Could you check a few things on this model? Use its own coordinates, in mm. Give positions to 0.01 mm unless a question says otherwise; leave off trailing zeros. Order: outer loops, then holes, each group sorted by start corner. A loop starts at its lowest first (then second) coordinate and runs counter-clockwise, first axis right, second up.
from build123d import *

# Parameters (mm, degrees)
SKETCH_1_R            = 3
SKETCH_1_R_2          = 7.5
SKETCH_1_R_3          = 6
EXTRUDE_1_DEPTH       = 4
CUT_EXTRUDE_START     = -10
CUT_EXTRUDE_2_DEPTH   = 10
CHAMFER_START         = -90.054290201
CHAMFER_2_OUTLINE_W   = 9.93243638
CHAMFER_2_OUTLINE_H   = 4
CHAMFER_2_DEPTH       = 0.082131492
CHAMFER_START_2       = -89.972158709
CHAMFER_2_2_OUTLINE_W = 9.93243638
CHAMFER_2_2_OUTLINE_H = 4
CHAMFER_2_2_DEPTH     = 1.179418362
FILLET_4_R            = 15
FILLET_5_R            = 10
CUT_EXTRUDE_6_DEPTH   = 10
FILLET_8_R            = 3


with BuildPart() as part:
    # 草图1 → 凸台-拉伸1 (new body)
    with BuildSketch(Plane.XY):
        with BuildLine():
            Line((-47.486974837, 85.838147942), (-18.140882386, -2.213296441))
            ThreePointArc((-18.140882386, -2.213296441), (-15.593099371, -5.678603485), (-11.5, -7))
            Line((-11.5, -7), (11.5, -7))
            ThreePointArc((11.5, -7), (16.545894038, -4.851695926), (18.494612442, 0.274584754))
            Line((18.494612442, 0.274584754), (14.988455233, 89.588395901))
            ThreePointArc((14.988455233, 89.588395901), (9.660960601, 100.474573642), (-1.973684211, 103.869585423))
            Line((-1.973684211, 103.869585423), (-39.315789474, 98.913056948))
            ThreePointArc((-39.315789474, 98.913056948), (-46.480167485, 94.299694277), (-47.486974837, 85.838147942))
        make_face()
        with Locations((11.5, 0)):
            Circle(SKETCH_1_R, mode=Mode.SUBTRACT)
        with Locations((-11.5, 0)):
            Circle(SKETCH_1_R, mode=Mode.SUBTRACT)
        with Locations((0, 89)):
            Circle(SKETCH_1_R_2, mode=Mode.SUBTRACT)
        with Locations((-38, 89)):
            Circle(SKETCH_1_R_3, mode=Mode.SUBTRACT)
    extrude(amount=EXTRUDE_1_DEPTH)

    # 草图3 → 切除-拉伸2 (cut)
    with BuildSketch(Plane.XY.offset(4).offset(CUT_EXTRUDE_START)):
        with BuildLine():
            Line((-30.07293559, 95.096035584), (-12.403974557, 97.441289229))
            ThreePointArc((-12.403974557, 97.441289229), (-8.018810771, 101.681191682), (-2.308312161, 103.825169261))
            Line((-2.308312161, 103.825169261), (-39.315789474, 98.913056948))
            ThreePointArc((-39.315789474, 98.913056948), (-34.182978636, 98.242853883), (-30.07293559, 95.096035584))
        make_face()
    extrude(amount=CUT_EXTRUDE_2_DEPTH, mode=Mode.SUBTRACT)

    # 倒角1
    # the kernel refuses this chamfer: 10 mm, written as the material it adds along each edge
    with BuildSketch(Plane(origin=(-30.07293559, 95.096035584, 0), x_dir=(-0.7655170404951253, 0.6434156205063604, 0), z_dir=(0, 0, 1))) as chamfer_1_piece_1:
        with BuildLine():
            Line((4.638446898, 0.2), (-5.12937843, -5.439456583))
            Line((-5.12937843, -5.439456583), (-5.277087929, -5.304616293))
            ThreePointArc((-5.277087929, -5.304616293), (-2.667716566, -2.625677211), (-0.147709499, 0.13484029))
            Line((-0.147709499, 0.13484029), (0.042920367, 0.195340324))
            ThreePointArc((0.042920367, 0.195340324), (2.321577959, -0.03141118), (4.595526531, 0.395340324))
            Line((4.595526531, 0.395340324), (4.638446898, 0.2))
        make_face()
    extrude(amount=4)

    # 倒角2: read off the stored shape, not the designer's step
    # 倒角2 outline → 倒角2 (cut)
    with BuildSketch(Plane(origin=(0, 0, 0), x_dir=(0.8432639594677478, 0.5374996694536441, 0), z_dir=(0.537499669453644, -0.8432639594677479, 0)).offset(CHAMFER_START)):
        with Locations((44.438996955, 2)):
            Rectangle(CHAMFER_2_OUTLINE_W, CHAMFER_2_OUTLINE_H)
    extrude(amount=CHAMFER_2_DEPTH, mode=Mode.SUBTRACT)

    # Chamfer 2 2 outline → Chamfer 2 2 (add)
    with BuildSketch(Plane(origin=(0, 0, 0), x_dir=(0.8432639594677478, 0.5374996694536441, 0), z_dir=(0.537499669453644, -0.8432639594677479, 0)).offset(CHAMFER_START_2)):
        with Locations((44.438996955, 2)):
            Rectangle(CHAMFER_2_2_OUTLINE_W, CHAMFER_2_2_OUTLINE_H)
    extrude(amount=CHAMFER_2_2_DEPTH)

    # 圆角4
    fillet_4_edges = [part.edges().sort_by_distance(p)[0] for p in [
        (-23.040343668, 96.029492385, 2),
        (-33.358562851, 97.857599065, 2),
        (-15.074033854, 97.086884333, 2),
    ]]
    fillet(fillet_4_edges, radius=FILLET_4_R)

    # 圆角5
    fillet_5_edges = [part.edges().sort_by_distance(p)[0] for p in [
        (-6.698368225, 102.425565605, 2),
    ]]
    fillet(fillet_5_edges, radius=FILLET_5_R)

    # 草图7 → 切除-拉伸6 (cut)
    with BuildSketch(Plane.XY.offset(4)):
        Polygon((3.302198464, 77), (-36.108751735, 77), (-15.314632791, 14.608313246), align=None)
        Polygon((10.185176898, 8), (7.961799494, 64.637023864), (-8.937918575, 8), align=None)
    extrude(amount=-CUT_EXTRUDE_6_DEPTH, mode=Mode.SUBTRACT)

    # 圆角8
    fillet_8_edges = [part.edges().sort_by_distance(p)[0] for p in [
        (7.961799494, 64.637023864, 2),
        (10.185176898, 8, 2),
        (-8.937918575, 8, 2),
        (3.302198464, 77, 2),
        (-15.314632791, 14.608313246, 2),
        (-36.108751735, 77, 2),
    ]]
    fillet(fillet_8_edges, radius=FILLET_8_R)


solid = part.part
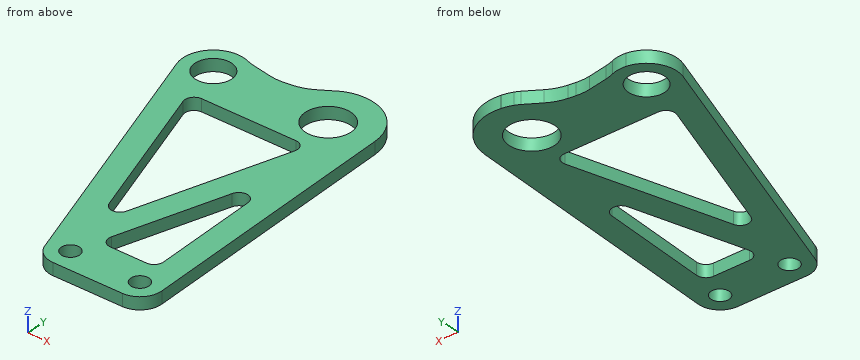
Item 1: Imagine slicing it at B-B on z = 1.8. Give the number of separate pieces and of enclosed holes in the cut face, then the cut area to 3 significant figures.
Findings:
separate pieces: 1
enclosed holes: 6
area: 3,310 mm2
Item 2: Please list where these lines run through material, in increasing order: line 1 along X through (y, z) = (84.5, 2.9); line 2 along Y through (x, z) = (-13, 0.85); line 3 along Y through (x, z) = (4.5, 0.2).
Findings:
line 1: x = -47.04 to -41.97, -34.03 to -6, 6 to 15.19
line 2: y = -6.84 to -2.6, 2.6 to 22.87, 77 to 98.44
line 3: y = -7 to 8, 49.23 to 83, 95 to 103.31
Item 3: For pin 1 (7 mm diameter, centred on x = 11.5, y = 0, fed in from +Z); pin 2 (1 mm diameter, centred on y = 34, z = 2, fed in from -X); pin 3 (2 mm diameter, centred on y = 36.5, z = 3.5, fed in from +X), each with a flat end and sliding along its axis, tell me the tip position at first contact or that it passes through.
Findings:
pin 1: stops at z = 4
pin 2: stops at x = -30.38
pin 3: stops at x = 17.11
Item 4: Imagine slicing it at A-A on x = -23. List the corners of the cut face in (y, z) for me.
Findings:
outline: (12.37, 0) - (37.67, 0) - (37.67, 4) - (12.37, 4) - close; (77, 0) - (96.21, 0) - (96.21, 4) - (77, 4) - close
Item 5: Imagine slicing it at C-C on x = -16. List the corners of the cut face in (y, z) for me.
Findings:
outline: (-5.36, 0) - (21.62, 0) - (21.62, 4) - (-5.36, 4) - close; (77, 0) - (97.16, 0) - (97.16, 4) - (77, 4) - close
